Geometry: final body of the model. Coordinates: model frame, mm. A direction names the side the tool comes from. Round coordinates to 2 decimals unless told otherwise and drop trailing zeros. Order: outer loops, then holes, each group sorted by start corner. A loop starts at its lowest first (then second) coordinate and runs counter-clockwise, first axis right, second up. Notation, with made-up numbers: (57, 43) -> (66, 43) arc R27 cw to (66, 75) -> close; hole circle Ø4 at (6.25, 14). An arc over 180 degrees is marked (long way). Put each result on its own line as item: value.
```python
from build123d import *

# Parameters (mm, degrees)
BOSS_EXTRUDE1_DEPTH = 55
BOSS_EXTRUDE3_DEPTH = 15
SKETCH4_W           = 190.013565595
SKETCH4_H           = 25
CUT_EXTRUDE1_DEPTH  = 36
SKETCH5_W           = 30
SKETCH5_H           = 30
CUT_EXTRUDE2_DEPTH  = 8
SKETCH6_W           = 72.414600628
SKETCH6_H           = 59.825353167
CUT_EXTRUDE3_DEPTH  = 40
SKETCH7_W           = 143.244471566
SKETCH7_H           = 49.658158813
CUT_EXTRUDE4_DEPTH  = 20
SKETCH8_W           = 131
SKETCH8_H           = 15
BOSS_EXTRUDE4_DEPTH = 55
FILLET1_R           = 8
CHAMFER1_SIZE       = 2


with BuildPart() as part:
    # Sketch1 → Boss-Extrude1 (new body)
    with BuildSketch(Plane.XY):
        with BuildLine():
            Line((-60.5, 65.5), (60.5, 65.5))
            ThreePointArc((60.5, 65.5), (74.642135624, 59.642135624), (80.5, 45.5))
            Line((80.5, 45.5), (80.5, -45.5))
            ThreePointArc((80.5, -45.5), (74.642135624, -59.642135624), (60.5, -65.5))
            Line((60.5, -65.5), (-60.5, -65.5))
            ThreePointArc((-60.5, -65.5), (-74.642135624, -59.642135624), (-80.5, -45.5))
            Line((-80.5, -45.5), (-80.5, 45.5))
            ThreePointArc((-80.5, 45.5), (-74.642135624, 59.642135624), (-60.5, 65.5))
        make_face()
        with BuildLine():
            Line((-65.5, 45.5), (-65.5, -45.5))
            ThreePointArc((-65.5, -45.5), (-62.571067812, -52.571067812), (-55.5, -55.5))
            Line((-55.5, -55.5), (55.5, -55.5))
            ThreePointArc((55.5, -55.5), (62.571067812, -52.571067812), (65.5, -45.5))
            Line((65.5, -45.5), (65.5, 45.5))
            ThreePointArc((65.5, 45.5), (62.571067812, 52.571067812), (55.5, 55.5))
            Line((55.5, 55.5), (-55.5, 55.5))
            ThreePointArc((-55.5, 55.5), (-62.571067812, 52.571067812), (-65.5, 45.5))
        make_face(mode=Mode.SUBTRACT)
    extrude(amount=BOSS_EXTRUDE1_DEPTH)

    # Sketch3 → Boss-Extrude3 (add)
    with BuildSketch(Plane(origin=(0, 0, 0), x_dir=(-1, 0, 0), z_dir=(0, 0, -1))):
        with BuildLine():
            Line((-80.5, 45.5), (-80.5, 65.5))
            ThreePointArc((-80.5, 65.5), (-74.642135624, 79.642135624), (-60.5, 85.5))
            Line((-60.5, 85.5), (60.5, 85.5))
            ThreePointArc((60.5, 85.5), (74.642135624, 79.642135624), (80.5, 65.5))
            Line((80.5, 65.5), (80.5, 45.5))
            ThreePointArc((80.5, 45.5), (74.642135624, 59.642135624), (60.5, 65.5))
            Line((60.5, 65.5), (-60.5, 65.5))
            ThreePointArc((-60.5, 65.5), (-74.642135624, 59.642135624), (-80.5, 45.5))
        make_face()
        with BuildLine():
            Line((80.5, -45.5), (80.5, -65.5))
            ThreePointArc((80.5, -65.5), (74.642135624, -79.642135624), (60.5, -85.5))
            Line((60.5, -85.5), (-60.5, -85.5))
            ThreePointArc((-60.5, -85.5), (-74.642135624, -79.642135624), (-80.5, -65.5))
            Line((-80.5, -65.5), (-80.5, -45.5))
            ThreePointArc((-80.5, -45.5), (-74.642135624, -59.642135624), (-60.5, -65.5))
            Line((-60.5, -65.5), (60.5, -65.5))
            ThreePointArc((60.5, -65.5), (74.642135624, -59.642135624), (80.5, -45.5))
        make_face()
    extrude(amount=-BOSS_EXTRUDE3_DEPTH)

    # Sketch4 → Cut-Extrude1 (cut)
    with BuildSketch(Plane.XY.offset(55)):
        with Locations((-0.225937653, -53)):
            Rectangle(SKETCH4_W, SKETCH4_H)
    extrude(amount=-CUT_EXTRUDE1_DEPTH, mode=Mode.SUBTRACT)

    # Sketch5 → Cut-Extrude2 (cut)
    with BuildSketch(Plane.XY.offset(19)):
        with Locations((0, -70.5)):
            Rectangle(SKETCH5_W, SKETCH5_H)
    extrude(amount=-CUT_EXTRUDE2_DEPTH, mode=Mode.SUBTRACT)

    # Sketch6 → Cut-Extrude3 (cut)
    with BuildSketch(Plane.XY.offset(55)):
        with Locations((-66.707300314, 45.412676584)):
            Rectangle(SKETCH6_W, SKETCH6_H)
    extrude(amount=-CUT_EXTRUDE3_DEPTH, mode=Mode.SUBTRACT)

    # Sketch7 → Cut-Extrude4 (cut)
    with BuildSketch(Plane.XY.offset(55)):
        with Locations((34.229554325, 70.329079407)):
            Rectangle(SKETCH7_W, SKETCH7_H)
    extrude(amount=-CUT_EXTRUDE4_DEPTH, mode=Mode.SUBTRACT)

    # Sketch8 → Boss-Extrude4 (add)
    with BuildSketch(Plane(origin=(0, 0, 0), x_dir=(-1, 0, 0), z_dir=(0, 0, -1))):
        with Locations((0, -5.5)):
            Rectangle(SKETCH8_W, SKETCH8_H)
    extrude(amount=-BOSS_EXTRUDE4_DEPTH)

    # Fillet1
    fillet1_edges = [part.edges().sort_by_distance(p)[0] for p in [
        (-65.5, -13, 27.5),
        (-65.5, 2, 27.5),
        (65.5, 2, 27.5),
        (65.5, -13, 27.5),
    ]]
    fillet(fillet1_edges, radius=FILLET1_R)

    # Chamfer1
    chamfer1_edges = [part.edges().sort_by_distance(p)[0] for p in [
        (80.5, 2.5, 55),
        (-80.5, -12.5, 55),
    ]]
    chamfer(chamfer1_edges, length=CHAMFER1_SIZE)


solid = part.part
```
1. Contact query for flat-ended pins moving along their axis: P1, Ø3, axis at y = 59, z = 20.5, coming from the -X side; P2, Ø20, axis at x = -45.5, y = -47, coming from the +Z side; P3, Ø16, axis at x = 16, y = 51, coming from the +Z side. Output: stop coordinate, or through.
Ans:
P1: x = -30.5
P2: z = 19
P3: z = 35
2. Draft query along Y for faces 1 (the face through (38, -65.5, 17)), 2 (the face through (80.5, -1, 26)), 3 (the face through (-1, -55.5, 9)), 4 (the face through (1, -13, 27)). Return one class per face: +Y half, -Y half, draft (parallel to the pull), parting line (faces both ways), or undercut.
Ans:
face 1: -Y half
face 2: draft
face 3: undercut
face 4: undercut
3. Cut plane A-A on x = -7. Return loops of the section in (y, z), and give its area (4 significant figures).
Ans:
outline: (-85.5, 0) -> (-55.5, 0) -> (-55.5, 11) -> (-85.5, 11) -> close; (-13, 0) -> (2, 0) -> (2, 55) -> (-13, 55) -> close; (55.5, 0) -> (85.5, 0) -> (85.5, 15) -> (65.5, 15) -> (65.5, 35) -> (55.5, 35) -> close
area: 1,805 mm²
4. Cut plane B-B on y = 30. Return loops of the section in (x, z), and give its area (3 significant figures).
Ans:
outline: (-80.5, 0) -> (-65.5, 0) -> (-65.5, 15) -> (-80.5, 15) -> close; (65.5, 0) -> (80.5, 0) -> (80.5, 53) -> (78.5, 55) -> (65.5, 55) -> close
area: 1,050 mm²
5. Set-up query: faces 5 (the face through (73, -40.5, 37)), 6 (the face through (63.219, 4.406, 27.885)), 7 (the face through (15, -67, 14)). Return all of +Z, -Z, +X, -X, +Y, -Y with unobstructed straight access to the full face (end or side cutting, diameter ignored); none if empty.
Ans:
face 5: +Z, +X, -X, -Y
face 6: +Z, -Z
face 7: +Z, -Y
6. Material intervals for probe 1 along Y at (x, z) = (32, 5); probe 2 along X at (y, z) = (25.5, 3); probe 3 along Y at (x, z) = (26, 29), sorted ascending.
Ans:
probe 1: -85.5 to -55.5, -13 to 2, 55.5 to 85.5
probe 2: -80.5 to -65.5, 65.5 to 80.5
probe 3: -13 to 2, 55.5 to 65.5
7. Cut plane D-D on z = 7.5. Return loops of the section in (x, y), and give its area (3 significant figures).
Ans:
outline: (-80.5, -65.5) arc R20 ccw to (-60.5, -85.5) -> (60.5, -85.5) arc R20 ccw to (80.5, -65.5) -> (80.5, 65.5) arc R20 ccw to (60.5, 85.5) -> (-60.5, 85.5) arc R20 ccw to (-80.5, 65.5) -> close; hole (-65.5, -45.5) arc R10 ccw to (-55.5, -55.5) -> (55.5, -55.5) arc R10 ccw to (65.5, -45.5) -> (65.5, -21) arc R8 ccw to (57.5, -13) -> (-57.5, -13) arc R8 ccw to (-65.5, -21) -> close; hole (-65.5, 10) arc R8 ccw to (-57.5, 2) -> (57.5, 2) arc R8 ccw to (65.5, 10) -> (65.5, 45.5) arc R10 ccw to (55.5, 55.5) -> (-55.5, 55.5) arc R10 ccw to (-65.5, 45.5) -> close
area: 14,800 mm²
8. Cut plane C-C on z = 29.5. Return loops of the section in (x, y).
Ans:
outline: (-80.5, -40.5) -> (-65.5, -40.5) -> (-65.5, -21) arc R8 cw to (-57.5, -13) -> (57.5, -13) arc R8 cw to (65.5, -21) -> (65.5, -40.5) -> (80.5, -40.5) -> (80.5, 45.5) arc R20 ccw to (60.5, 65.5) -> (-30.5, 65.5) -> (-30.5, 55.5) -> (55.5, 55.5) arc R10 cw to (65.5, 45.5) -> (65.5, 10) arc R8 cw to (57.5, 2) -> (-57.5, 2) arc R8 cw to (-65.5, 10) -> (-65.5, 15.5) -> (-80.5, 15.5) -> close
